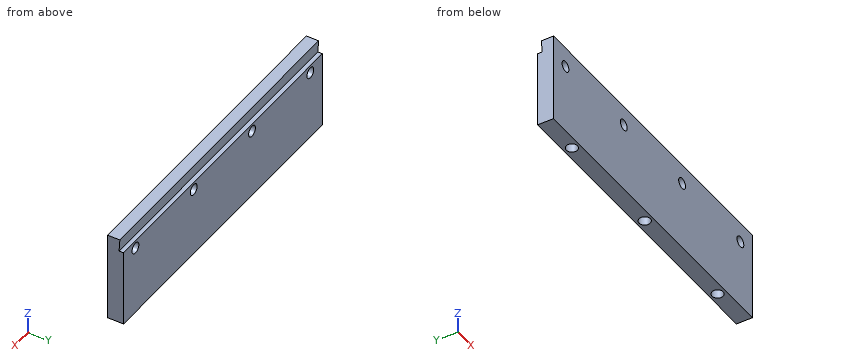
from build123d import *

# Parameters (mm, degrees)
F0_W     = 190.5
F0_H     = 54.1147
F1_DEPTH = 9.525
F3_D     = 6.5278
F5_DEPTH = 190.501
F7_D     = 6.7564
F7_DEPTH = 12.7
F7_TIP   = 2.0298273432


with BuildPart() as f1:
    # F0 (on Front) → F1 (new body)
    with BuildSketch(Plane.XZ):
        with Locations((95.25, 27.05735)):
            Rectangle(F0_W, F0_H)
    extrude(amount=F1_DEPTH)

    # F3 (through all)
    with Locations(Plane.XZ.offset(9.525)):
        with Locations((11.46175, 41.97985), (67.34175, 41.97985), (123.20905, 41.97985), (179.08905, 41.97985)):
            Hole(F3_D / 2)

    # F4 (on face) → F5 (cut, through all)
    with BuildSketch(Plane.YZ.offset(190.5)):
        Polygon((0, 54.1147), (-2.2098, 54.1147), (-2.6924, 46.6344), (0, 46.6344), align=None)
    extrude(amount=-F5_DEPTH, mode=Mode.SUBTRACT)

    # F7
    with Locations(Plane(origin=(0, 0, 0), x_dir=(1, 0, 0), z_dir=(0, 0, -1))):
        with Locations((25.13965, 4.7969794832), (94.92615, 4.7969794832), (164.77615, 4.7969794832)):
            Hole(F7_D / 2, depth=F7_DEPTH)
            with Locations((0, 0, -(F7_DEPTH + F7_TIP / 2))):  # 118° drill point
                Cone(0, F7_D / 2, F7_TIP, mode=Mode.SUBTRACT)


solid = f1.part
Build history of the part. All positions in model axes, mm. Round coordinates to 2 decimals unless told otherwise and drop trailing zeros. Write each loop counter-clockwise with the first axis right and the second up, starting at its lowest first coordinate (ties: lowest second). Pieces come first, ordered by that corner, then holes. Notation, with made-up numbers: M 16.25,24.25 L 37.25,24.25 A12 cw 37.25,40.25 Z; hole C 72,15 d9. An arc over 180 degrees is marked long. Answer as a JSON object with one key per item and string values. Group by question number.
(1) Cut at A-A (x = 129). Give the cut face in (y, z) (3 decimals).
(2) Drill centre lines: L1, parallel to X at y = -4.5, z = 5; L2, parallel to Y at x = 94.5, z = 4 (3 decimals); L3, parallel to X at y = -4.75, z = 5.5. Where is each one in solid material? Low to high.
(3) Cut at B-B (z = 3). Give the cut face in (x, y) (3 decimals).
(4) Flat gauge pins, fed straight in: pin 1 (2 mm diameter, centred on x = 105, z = 43.5, fed in from +Y); pin 2 (5 mm diameter, centred on x = 123.21, z = 41.98, fed in from -Y); pin 3 (5.5 mm diameter, centred on x = 25.14, y = -4.8, fed in from -Z); pin 4 (1.3 mm diameter, centred on x = 113.5, y = -1, fed in from +Z). Where does each tip first touch, or does it go through?
Responses:
{
 "1": {"outline": "M -9.525,0 L 0,0 L 0,46.634 L -2.692,46.634 L -2.21,54.115 L -9.525,54.115 Z"},
 "2": {"L1": "x = 0 to 21.77, 28.5 to 91.56, 98.29 to 161.41, 168.14 to 190.5", "L2": "y = -9.525 to -8.148, -1.446 to 0", "L3": "x = 0 to 21.76, 28.52 to 91.55, 98.3 to 161.4, 168.15 to 190.5"},
 "3": {"outline": "M 0,-9.525 L 190.5,-9.525 L 190.5,0 L 0,0 Z; hole C 25.14,-4.797 d6.756; hole C 94.926,-4.797 d6.756; hole C 164.776,-4.797 d6.756"},
 "4": {"pin 1": "stops at y = 0", "pin 2": "passes through", "pin 3": "stops at z = 13.08", "pin 4": "stops at z = 46.63"}
}
